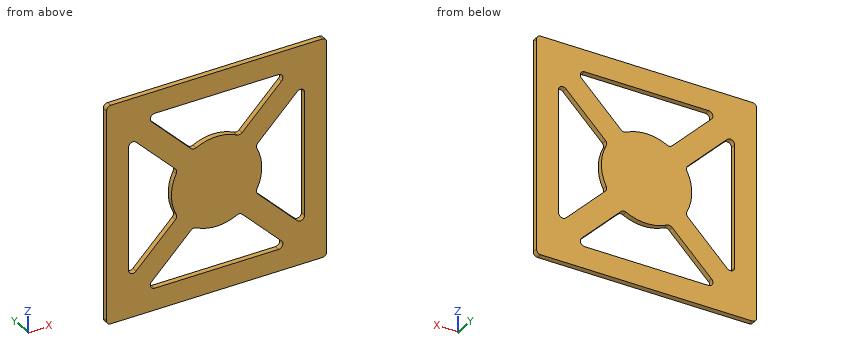
```python
from build123d import *

# Parameters (mm, degrees)
SKETCH1_W           = 500
SKETCH1_H           = 500
BOSS_EXTRUDE1_DEPTH = 12
CUT_EXTRUDE1_DEPTH  = 12
FILLET1_R           = 10


with BuildPart() as part:
    # Sketch1 → Boss-Extrude1 (new body)
    with BuildSketch(Plane(origin=(0, 0, 0), x_dir=(1, 0, 0), z_dir=(0, 1, 0))):
        Rectangle(SKETCH1_W, SKETCH1_H)
    extrude(amount=BOSS_EXTRUDE1_DEPTH)

    # Sketch2 → Cut-Extrude1 (cut)
    with BuildSketch(Plane(origin=(0, 12, 0), x_dir=(1, 0, 0), z_dir=(0, 1, 0))):
        with BuildLine():
            Line((-200, 164.644660941), (-88.091394352, 52.736055293))
            ThreePointArc((-88.091394352, 52.736055293), (-102.670274602, 0), (-88.091394352, -52.736055293))
            Line((-88.091394352, -52.736055293), (-200, -164.644660941))
            Line((-200, -164.644660941), (-200, 164.644660941))
        make_face()
        with BuildLine():
            Line((164.644660941, 200), (52.736055293, 88.091394352))
            ThreePointArc((52.736055293, 88.091394352), (0, 102.670274602), (-52.736055293, 88.091394352))
            Line((-52.736055293, 88.091394352), (-164.644660941, 200))
            Line((-164.644660941, 200), (164.644660941, 200))
        make_face()
        with BuildLine():
            Line((200, 164.644660941), (88.091394352, 52.736055293))
            ThreePointArc((88.091394352, 52.736055293), (102.670274602, 0), (88.091394352, -52.736055293))
            Line((88.091394352, -52.736055293), (200, -164.644660941))
            Line((200, -164.644660941), (200, 164.644660941))
        make_face()
        with BuildLine():
            Line((-164.644660941, -200), (164.644660941, -200))
            Line((164.644660941, -200), (52.736055293, -88.091394352))
            ThreePointArc((52.736055293, -88.091394352), (0, -102.670274602), (-52.736055293, -88.091394352))
            Line((-52.736055293, -88.091394352), (-164.644660941, -200))
        make_face()
    extrude(amount=-CUT_EXTRUDE1_DEPTH, mode=Mode.SUBTRACT)

    # Fillet1
    fillet1_edges = [part.edges().sort_by_distance(p)[0] for p in [
        (-200, 6, 164.644660941),
        (-200, 6, -164.644660941),
        (-88.091394352, 6, -52.736055293),
        (-88.091394352, 6, 52.736055293),
        (-164.644660941, 6, -200),
        (164.644660941, 6, -200),
        (52.736055293, 6, -88.091394352),
        (-52.736055293, 6, -88.091394352),
        (52.736055293, 6, 88.091394352),
        (164.644660941, 6, 200),
        (-164.644660941, 6, 200),
        (-52.736055293, 6, 88.091394352),
        (88.091394352, 6, 52.736055293),
        (88.091394352, 6, -52.736055293),
        (200, 6, -164.644660941),
        (200, 6, 164.644660941),
        (-250, 6, -250),
        (250, 6, -250),
        (250, 6, 250),
        (-250, 6, 250),
    ]]
    fillet(fillet1_edges, radius=FILLET1_R)


solid = part.part
```
The listing builds one solid part. Answer for the finished solid, in the listing's coordinates (mm). Round coordinates to 2 decimals unless told otherwise and drop trailing zeros. Order: outer loops, then holes, each group sorted by start corner. A loop starts at its lowest first (then second) coordinate and runs counter-clockwise, first axis right, second up. Notation, with made-up numbers: (-1.75, -29) - (8.25, -29) arc R14 cw to (8.25, -13) - close; hole circle Ø6 at (5, 74). An arc over 180 degrees is marked (long way). Put each result on its own line as item: value. Start each with the question number.
(1) Find section A-A (x = -170). Give the vertices of the cut face in (y, z).
(2) Straight lines are drawn through the part: probe 1 along Z at (x, y) = (-144.5, 8); probe 2 along X at (y, z) = (9.5, 14.5); probe 3 along X at (y, z) = (11, 73). For each, find the intervals that lie inside material, in ascending order. Write a range as from..to.
(3) Find section C-C (z = -126.5). Give the vertices of the cut face in (x, y), plus the area to 3 significant figures.
(4) Find section D-D (y = 5.75). State how many separate pieces and enclosed holes the cut face has, plus the area to 3 significant figures.
(5) Find section B-B (x = -67.5). Give the vertices of the cut face in (y, z).
Reply:
1. outline: (0, -250) - (12, -250) - (12, -134.64) - (0, -134.64) - close; (0, 134.64) - (12, 134.64) - (12, 250) - (0, 250) - close
2. probe 1: -250..-199.17, -179.86..-109.14, 109.14..179.86, 199.17..250
2. probe 2: -250..-200, -101.64..101.64, 200..250
2. probe 3: -250..-200, -108.36..108.36, 200..250
3. outline: (-250, 0) - (-200, 0) - (-200, 12) - (-250, 12) - close; (-161.86, 0) - (-91.14, 0) - (-91.14, 12) - (-161.86, 12) - close; (91.14, 0) - (161.86, 0) - (161.86, 12) - (91.14, 12) - close; (200, 0) - (250, 0) - (250, 12) - (200, 12) - close
3. area: 2,900 mm^2
4. separate pieces: 1
4. enclosed holes: 4
4. area: 158,000 mm^2
5. outline: (0, -250) - (12, -250) - (12, -200) - (0, -200) - close; (0, -102.86) - (12, -102.86) - (12, 102.86) - (0, 102.86) - close; (0, 200) - (12, 200) - (12, 250) - (0, 250) - close
